Print and shaded views of the part. All mm, measured from the part's lowest x, y and z. Round coordinates to 2 decimals unless told otherwise and drop trailing zeros. Loops run counter-clockwise (first coordinate to the right, second up) from the corner with the lowest first, then second, coordinate; pieces in that order, holes last. Notation, with made-up numbers: (44, 49) -> (58, 49) arc R17 ccw to (58, 53) -> close; hole circle Ø11 at (59.5, 25). An arc over 180 degrees is marked (long way). Answer as CSV lines item,"result".
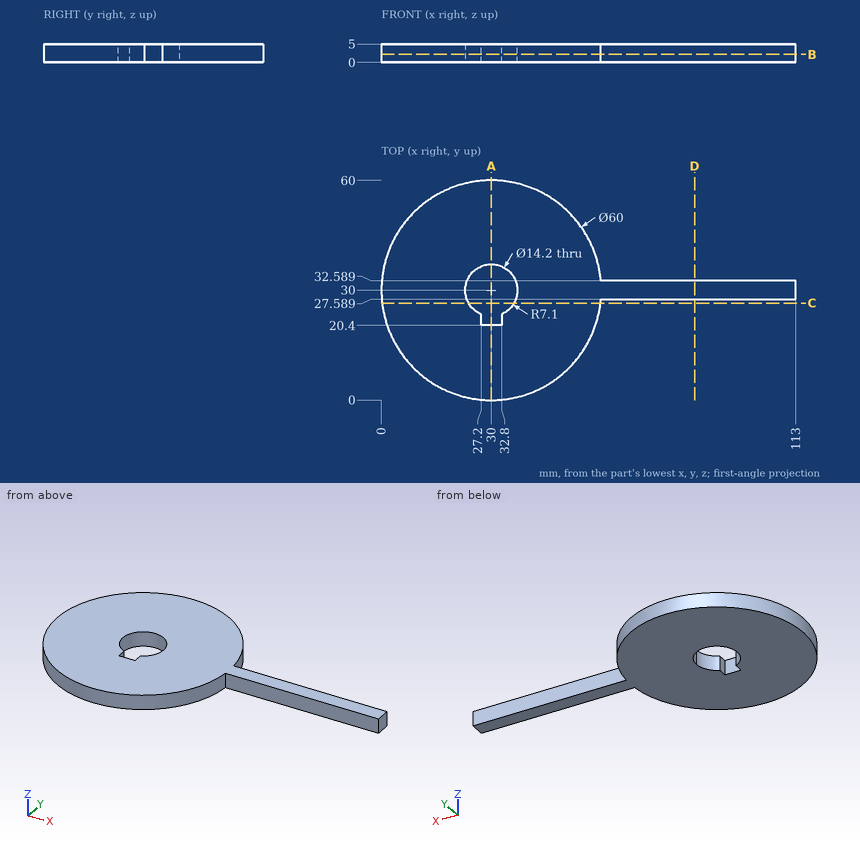
Q1. Slice it at B-B, the plane z = 2.15. Give the cut face in (x, y), and give its area (3 significant figures).
Results:
outline,"(59.89, 32.59) arc R30 ccw (long way) to (59.9, 27.59) -> (113, 27.59) -> (113, 32.59) -> close; hole (27.2, 20.4) -> (32.8, 20.4) -> (32.8, 23.48) arc R7.1 ccw (long way) to (27.2, 23.48) -> close"
area,"2,920 mm2"
Q2. Probe L1, parallel to Y at x = 30, z = 3.1; L2, parallel to Y at x = 65, z = 4.8; L3, parallel to Y at x = 26.5, z = 2.7 (1 decimal). List the from-to ranges inside material, lowest first. Write a range as [from, to].
Results:
L1,"[0, 20.4], [37.1, 60]"
L2,"[27.59, 32.59]"
L3,"[0.2, 23.8], [36.2, 59.8]"
Q3. Slice it at A-A, the plane x = 30. Give the cut face in (y, z).
Results:
outline,"(0, 0) -> (20.4, 0) -> (20.4, 5) -> (0, 5) -> close; (37.1, 0) -> (60, 0) -> (60, 5) -> (37.1, 5) -> close"
Q4. Slice it at D-D, the plane x = 85.5. Give the cut face in (y, z), and give its area (3 significant figures).
Results:
outline,"(27.59, 0) -> (32.59, 0) -> (32.59, 5) -> (27.59, 5) -> close"
area,"25.0 mm2"
Q5. Slice it at C-C, the plane y = 26.5. Give the cut face in (x, z) (1 decimal), and give its area (3 significant figures).
Results:
outline,"(0.2, 0) -> (23.8, 0) -> (23.8, 5) -> (0.2, 5) -> close; (36.2, 0) -> (59.8, 0) -> (59.8, 5) -> (36.2, 5) -> close"
area,"236 mm2"
Q6. Drop flat-ended pins along their axis: pin 1 Ø1.5 at (y, z) = (21.5, 3.5) entering from -X; pin 2 Ø8.5 at (x, y) = (30, 30) entering from +Z; pin 3 Ø2.5 at (y, z) = (22, 3) entering from +X; pin 4 Ø2 at (y, z) = (24, 2.5) entering from +X. Give the stop position or say it passes through.
Results:
pin 1,"x = 1.02"
pin 2,"through"
pin 3,"x = 59.23"
pin 4,"x = 59.58"
